Autodesk Inventor part; units mm, degrees
ref_plane "YZ Plane" through (0, 0, 0) normal (1, 0, 0) x (0, 1, 0)
ref_plane "XZ Plane" through (0, 0, 0) normal (0, 1, 0) x (-1, 0, 0)
ref_plane "XY Plane" through (0, 0, 0) normal (0, 0, 1) x (1, 0, 0)
sketch "Sketch1" plane through (0, 0, 0) normal (0, 1, 0) x (-1, 0, 0)
  line L0 (-5.3975, -59.69) -> (5.3975, -59.69)
  line L1 (15.5575, -49.53) -> (15.5575, 59.69)
  line L2 (15.5575, 59.69) -> (-15.5575, 59.69)
  line L3 (-15.5575, 59.69) -> (-15.5575, -49.53)
  line L4 (-15.5575, -59.69) -> (15.5575, 59.69) construction
  line L5 (15.5575, -59.69) -> (-15.5575, 59.69) construction
  arc A0 (5.3975, -59.69) -> (15.5575, -49.53) centre (5.3975, -49.53) ccw
  arc A1 (-15.5575, -49.53) -> (-5.3975, -59.69) centre (-5.3975, -49.53) ccw
  circle A2 centre (0, 34.29) radius 7.9375
  point P0 (0, 0)
  dimension "d0" = 119.38
  dimension "d1" = 31.115
  dimension "d2" = 10.16
  dimension "d3" = 15.875
  dimension "d4" = 25.4
extrude "Extrusion1" add sketch "Sketch1" along normal blind 37.719
sketch "Sketch2" plane through (0, 37.719, 0) normal (0, 1, 0) x (1, 0, 0)
  line L0 (5.3975, 59.69) -> (-5.3975, 59.69)
  point P0 (0, 0)
  point P1 (0, 34.29)
  dimension "d7" = 25.4
hole "Hole1" at (0, 37.719, -34.29) direction (0, -1, 0) diameter 12.7 end through all
hole "Hole3" at (0.3897, 17.4911, 59.69) direction (0, 0, -1) diameter 6.35 depth 12.7 tip angle 118
hole "Hole4" at (-15.5575, 17.5708, -16.4401) direction (1, 0, 0) diameter 6.35 depth 12.7 tip angle 118
hole "Hole5" at (15.5575, 16.4302, -30.8144) direction (-1, 0, 0) diameter 6.35 depth 12.7 tip angle 118
properties part number "Fixture_Base"
Build history of the part. All positions in model axes, mm. A direction names the side the tool comes from. Coordinates: 2 decimals unless noted, no trailing zeros. Order: outer loops, then holes, each group sorted by start corner. A loop starts at its lowest first (then second) coordinate and runs counter-clockwise, first axis right, second up. Notation, with made-up numbers: (44.25, -30.5) -> (81.25, -30.5) arc R37 ccw to (81.25, 6.5) -> close; hole circle Ø6 at (88, -31). An arc over 180 degrees is marked (long way). Answer in a Markdown table with one row per item. Add a question column.
Q1. Band-saw the part on B-B, the plane z = 34.29. List the corners of the cut face in (x, y), then the cut area to 3 significant figures.
Q2. Drop flat-ended pins along their axis: pin 1 (5.5 mm diameter, centred on x = 0.39, y = 17.49, fed in from +Z); pin 2 (14.5 mm diameter, centred on x = 0, z = 34.29, fed in from -Y); pin 3 (8 mm diameter, centred on x = -11, y = 24.5, fed in from -Z). Give the stop position or say it passes through.
Q3. Wall check: line 1 along Z through (x, y) = (0, 12); line 2 along Z through (x, y) = (-4.5, 5.5); line 3 along X through (y, z) = (17.5, 50). Give the ranges that are in metal, low to high. Write a range as [from, to].
Q4. Which spindle directions (+Z, -Z, +X, -X, +Y, -Y) get a long thin tool onto all of the face, cutting with end or side? Do faces 1 (the face through (-9.12, 17.43, -19.61)), 2 (the face through (-0.56, 14.46, 53.25)), 3 (the face through (-15.558, 19, 4)). Say none if no direction does.
Q5. Band-saw the part on A-A, the plane y = 9. Give the number of separate pieces and of enclosed holes in the cut face, then the cut area to 3 significant figures.
Q6. Band-saw the part on C-C, the plane x = 10.5. List the corners of the cut face in (y, z) (3 decimals).
Q7. Mould opens along Y. For faces 4 (the face through (0, 0, 1)), 5 (the face through (0, 37.719, 1)), 6 (the face through (10.53, 16.291, -27.642)), 7 (the face through (1.03, 18.6, 26.42)) say: +Y half, -Y half, draft (parallel to the pull), parting line (faces both ways), or undercut.
Answers follow:
| question | item | result |
|---|---|---|
| 1 | outline | (-15.56, 0) -> (-7.94, 0) -> (-7.94, 37.72) -> (-15.56, 37.72) -> close; (7.94, 0) -> (15.56, 0) -> (15.56, 37.72) -> (7.94, 37.72) -> close |
| 1 | area | 575 mm^2 |
| 2 | pin 1 | z = 46.74 |
| 2 | pin 2 | through |
| 2 | pin 3 | z = -59.56 |
| 3 | line 1 | [-59.69, -40.64], [-27.94, 26.35], [42.23, 59.69] |
| 3 | line 2 | [-59.69, -38.77], [-29.81, 27.75], [40.83, 59.69] |
| 3 | line 3 | [-15.56, -2.79], [3.56, 15.56] |
| 4 | face 1 | -X |
| 4 | face 2 | +Z |
| 4 | face 3 | +Z, -Z, -X, +Y, -Y |
| 5 | separate pieces | 1 |
| 5 | enclosed holes | 2 |
| 5 | area | 3,350 mm^2 |
| 6 | outline | (0, -58.316) -> (37.719, -58.316) -> (37.719, 59.69) -> (0, 59.69) -> close; hole circle Ø6.35 at (16.43, -30.814) |
| 7 | face 4 | -Y half |
| 7 | face 5 | +Y half |
| 7 | face 6 | undercut |
| 7 | face 7 | draft |
